For this review, take the finished solid that the model builds, in its own axes (mm). Coordinates: 2 decimals unless noted, no trailing zeros. Loops run counter-clockwise (first coordinate to the right, second up) from the corner with the lowest first, then second, coordinate; pieces in that order, holes last. Notation, with made-up numbers: (55.5, 41.25) -> (78.5, 41.25) arc R8 ccw to (78.5, 48.25) -> close; hole circle Ø1 at (34, -38.75). An arc over 180 degrees is marked (long way). Use a Markdown table: item, result.
from build123d import *

# Parameters (mm, degrees)
BOSS_EXTRUDE1_DEPTH = 7.62
SKETCH5_W           = 7.62
SKETCH5_H           = 15.24
CUT_EXTRUDE5_DEPTH  = 8.62


with BuildPart() as part:
    # Sketch1 → Boss-Extrude1 (new body)
    with BuildSketch(Plane(origin=(0, 0, 0), x_dir=(1, 0, 0), z_dir=(0, 1, 0))):
        with BuildLine():
            Line((-88.9, 0), (-88.9, 76.2))
            ThreePointArc((-88.9, 76.2), (0, 165.1), (88.9, 76.2))
            Line((88.9, 76.2), (88.9, 0))
            ThreePointArc((88.9, 0), (0, -88.9), (-88.9, 0))
        make_face()
    extrude(amount=BOSS_EXTRUDE1_DEPTH)

    # Sketch5 → Cut-Extrude5 (cut, through all)
    with BuildSketch(Plane(origin=(0, 7.62, 0), x_dir=(1, 0, 0), z_dir=(0, 1, 0))):
        with Locations((80.01, -11.43)):
            Rectangle(SKETCH5_W, SKETCH5_H)
        with Locations((-80.01, -11.43)):
            Rectangle(SKETCH5_W, SKETCH5_H)
        with Locations((-80.01, 87.63)):
            Rectangle(SKETCH5_W, SKETCH5_H)
        with Locations((80.01, 87.63)):
            Rectangle(SKETCH5_W, SKETCH5_H)
        with Locations((80.01, 38.1)):
            Rectangle(SKETCH5_W, SKETCH5_H)
        with Locations((-80.01, 38.1)):
            Rectangle(SKETCH5_W, SKETCH5_H)
    extrude(amount=-CUT_EXTRUDE5_DEPTH, mode=Mode.SUBTRACT)


solid = part.part
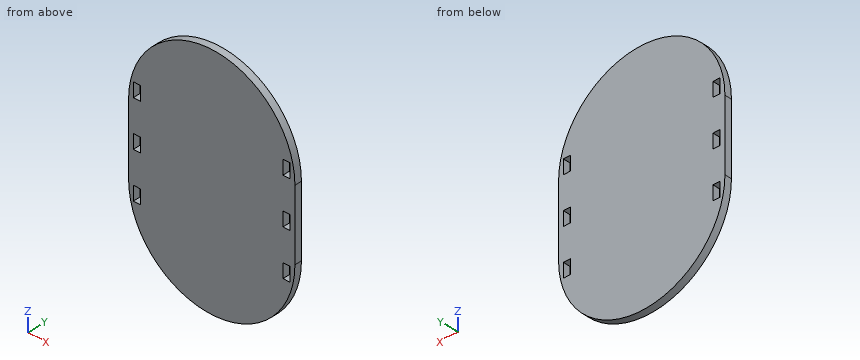
(1) Take a section at C-C on x = 53.5. Write out the cut boundary in (y, z).
Found:
| item | result |
|---|---|
| outline | (0, -147.2) -> (7.62, -147.2) -> (7.62, 71) -> (0, 71) -> close |
(2) Take a section at D-D on z = 25. Write out the cut boundary in (x, y), plus the area to 3 significant figures.
Found:
| item | result |
|---|---|
| outline | (-85.31, 0) -> (85.31, 0) -> (85.31, 7.62) -> (-85.31, 7.62) -> close |
| area | 1,300 mm^2 |
(3) Take a section at B-B on z = -84. Write out the cut boundary in (x, y).
Found:
| item | result |
|---|---|
| outline | (-88.56, 0) -> (-83.82, 0) -> (-83.82, 7.62) -> (-88.56, 7.62) -> close; (-76.2, 0) -> (76.2, 0) -> (76.2, 7.62) -> (-76.2, 7.62) -> close; (83.82, 0) -> (88.56, 0) -> (88.56, 7.62) -> (83.82, 7.62) -> close |
(4) For pin 1 Ø4 at (x, y) = (78.5, 3.5) entering from -Z; pin 2 Ø4 at (x, y) = (42, 2) entering from -Z; pin 3 Ø2.5 at (y, z) = (2.5, 15) entering from -X, all flat-tipped, find the tip position at first contact; note any pin that passes through.
Found:
| item | result |
|---|---|
| pin 1 | stops at z = -121.49 |
| pin 2 | stops at z = -155.59 |
| pin 3 | stops at x = -87.83 |
(5) Take a section at A-A on y = 3.25. Write out the cut boundary in (x, z), plus the area to 3 significant figures.
Found:
| item | result |
|---|---|
| outline | (-88.9, -76.2) arc R88.9 ccw to (88.9, -76.2) -> (88.9, 0) arc R88.9 ccw to (-88.9, 0) -> close; hole (-83.82, -95.25) -> (-76.2, -95.25) -> (-76.2, -80.01) -> (-83.82, -80.01) -> close; hole (-83.82, -45.72) -> (-76.2, -45.72) -> (-76.2, -30.48) -> (-83.82, -30.48) -> close; hole (-83.82, 3.81) -> (-76.2, 3.81) -> (-76.2, 19.05) -> (-83.82, 19.05) -> close; hole (76.2, -95.25) -> (83.82, -95.25) -> (83.82, -80.01) -> (76.2, -80.01) -> close; hole (76.2, -45.72) -> (83.82, -45.72) -> (83.82, -30.48) -> (76.2, -30.48) -> close; hole (76.2, 3.81) -> (83.82, 3.81) -> (83.82, 19.05) -> (76.2, 19.05) -> close |
| area | 37,700 mm^2 |
(6) For line 1 along X through (y, z) = (2.25, -34); line 2 along X through (y, z) = (5.5, -81); line 3 along Z through (x, y) = (78.5, 2.5), list the stretches that pass through material, from the lowest coordinate up.
Found:
| item | result |
|---|---|
| line 1 | x = -88.9 to -83.82, -76.2 to 76.2, 83.82 to 88.9 |
| line 2 | x = -88.77 to -83.82, -76.2 to 76.2, 83.82 to 88.77 |
| line 3 | z = -117.92 to -95.25, -80.01 to -45.72, -30.48 to 3.81, 19.05 to 41.72 |
